```python
from build123d import *

# Parameters (mm, degrees)
F1_DEPTH    = 30
F2_W        = 1278
F2_H        = 510
F3_DEPTH    = 28
F4_W        = 500
F4_H        = 400
F5_DEPTH    = 300
F6_T        = 2
F6_T3_DEPTH = 34
F6_T5_DEPTH = 404
F6_T7_DEPTH = 504
F6_T9_DEPTH = 32
F7_R        = 50
F8_R        = 25
F9_DEPTH    = 2
F10_R       = 15
F10_R_2     = 20
F11_DEPTH   = 30
F12_W       = 510
F12_H       = 2
F13_DEPTH   = 5
F14_W       = 510
F14_H       = 2
F15_ANGLE   = 90
F16_W       = 2
F16_H       = 510
F17_DEPTH   = 10
F19_DEPTH   = 400
F20_R       = 150
F21_W       = 30
F21_H       = 30
F22_DEPTH   = 850
F23_W       = 30
F23_H       = 30
F24_DEPTH   = 1080
F25_W       = 30
F25_H       = 30
F26_DEPTH   = 480
F28_DEPTH   = 2


# Not quite as in the source:
# - a shell that OpenCascade refuses in one call is made with other operations: the cavity is built on its own and cut out


with BuildPart() as f1:
    # F0 (on Top) → F1 (new body)
    with BuildSketch(Plane.XY):
        Polygon((0, 690), (0, 0), (1280, 0), (1280, 725), (100, 725), (100, 690), align=None)
    extrude(amount=F1_DEPTH)

    # F2 (on face) → F3 (cut)
    with BuildSketch(Plane.XY.offset(30)):
        with Locations((641, 285)):
            Rectangle(F2_W, F2_H)
    extrude(amount=-F3_DEPTH, mode=Mode.SUBTRACT)

    # F4 (on face) → F5 (join)
    with BuildSketch(Plane(origin=(0, 0, 0), x_dir=(1, 0, 0), z_dir=(0, 0, -1))):
        with Locations((370, -285)):
            Rectangle(F4_W, F4_H)
    extrude(amount=F5_DEPTH)

    # F6: shell of thickness 2, made by hand


with BuildPart() as f6_core1:
    # F6_t2: copy of F1
    add(f1.part)

    # the walls: a layer under each face that stays
    f6_faces = [f6_core1.faces().sort_by_distance(p)[0] for p in [
        (0, 345, 15),
        (50, 690, 15),
        (640, 0, 15),
        (640, 362.5, 0),
        (213.3333333333, 604.1666666667, 30),
        (100, 707.5, 15),
        (1280, 604.1666666667, 25),
        (690, 725, 15),
        (620, 285, -150),
        (370, 485, -150),
        (120, 285, -150),
        (370, 85, -150),
        (641, 540, 16),
        (2, 285, 16),
        (641, 30, 16),
        (370, 285, -300),
    ]]
    thicken(f6_faces, amount=-F6_T, mode=Mode.SUBTRACT)

    # F6_s4 → F6_t3 (cut)
    with BuildSketch(Plane.XY.offset(-2)):
        Polygon((99.98, 690.02), (100, 688), (102, 688), (102, 690), align=None)
    extrude(amount=F6_T3_DEPTH, mode=Mode.SUBTRACT)

    # F6_s6 → F6_t5 (cut)
    with BuildSketch(Plane.XZ.offset(-487)):
        Polygon((620.02, -0.02), (620, 2), (618, 2), (618, 0), align=None)
        Polygon((119.98, -0.02), (120, 2), (122, 2), (122, 0), align=None)
    extrude(amount=F6_T5_DEPTH, mode=Mode.SUBTRACT)

    # F6_s8 → F6_t7 (cut)
    with BuildSketch(Plane.YZ.offset(118)):
        Polygon((485.02, -0.02), (485, 2), (483, 2), (483, 0), align=None)
        Polygon((84.98, -0.02), (85, 2), (87, 2), (87, 0), align=None)
    extrude(amount=F6_T7_DEPTH, mode=Mode.SUBTRACT)

    # F6_s10 → F6_t9 (cut)
    with BuildSketch(Plane.XY):
        Polygon((2.02, 539.98), (2, 542), (0, 542), (0, 540), align=None)
        Polygon((2.02, 30.02), (0, 30), (0, 28), (2, 28), align=None)
    extrude(amount=F6_T9_DEPTH, mode=Mode.SUBTRACT)


with BuildPart() as f1_1:
    add(f1.part)

    # what is left inside the walls is the cavity
    f6_cavity = [f6_core1.part.solids().sort_by_distance(p)[0] for p in [
        (640, 10.666667, 2.02),
        (640, 602.333333, 27.98),
        (370, 351, -297.98),
    ]]
    add(f6_cavity, mode=Mode.SUBTRACT)

    # F7
    f7_edges = [f1_1.edges().sort_by_distance(p)[0] for p in [
        (122, 483, -148),
        (618, 483, -148),
        (122, 87, -148),
        (618, 87, -148),
        (618, 285, -298),
        (370, 483, -298),
        (122, 285, -298),
        (370, 87, -298),
        (120, 85, -150),
        (370, 85, -300),
        (620, 85, -150),
        (620, 285, -300),
        (620, 485, -150),
        (370, 485, -300),
        (120, 485, -150),
        (120, 285, -300),
    ]]
    fillet(f7_edges, radius=F7_R)

    # F8 (on face) → F9 (cut, through all)
    with BuildSketch(Plane.XY.offset(-298)):
        with Locations((488, 353)):
            Circle(F8_R)
    extrude(amount=-F9_DEPTH, mode=Mode.SUBTRACT)

    # F10 (on face) → F11 (cut, through all)
    with BuildSketch(Plane.XY.offset(30)):
        with Locations((550, 632.5)):
            Circle(F10_R)
        with Locations((370, 632.5)):
            Circle(F10_R)
        with Locations((190, 632.5)):
            Circle(F10_R_2)
    extrude(amount=-F11_DEPTH, mode=Mode.SUBTRACT)

    # F12 (on face) → F13 (join)
    with BuildSketch(Plane.YZ.offset(1280)):
        with Locations((285, 1)):
            Rectangle(F12_W, F12_H)
    extrude(amount=F13_DEPTH)

    # F14 (on face) → F15 (revolve)
    with BuildSketch(Plane.YZ.offset(1285)):
        with Locations((285, 1)):
            Rectangle(F14_W, F14_H)
    revolve(axis=Axis((1285, 285, 0), (0, 1, 0)), revolution_arc=F15_ANGLE)

    # F16 (on face) → F17 (join)
    with BuildSketch(Plane(origin=(0, 0, 0), x_dir=(1, 0, 0), z_dir=(0, 0, -1))):
        with Locations((1286, -285)):
            Rectangle(F16_W, F16_H)
    extrude(amount=F17_DEPTH)

    # F18 (on face) → F19 (join)
    with BuildSketch(Plane.XY.offset(30)):
        Polygon((1278, 540), (1280, 540), (1280, 725), (100, 725), (100, 690), (0, 690), (0, 0), (2, 0), (2, 688), (102, 688), (102, 723), (1278, 723), align=None)
    extrude(amount=F19_DEPTH)

    # F20
    f20_edges = [f1_1.edges().sort_by_distance(p)[0] for p in [
        (1279, 540, 430),
        (1, 0, 430),
    ]]
    fillet(f20_edges, radius=F20_R)

    # F21 (on face) → F22 (join)
    with BuildSketch(Plane(origin=(0, 0, 0), x_dir=(1, 0, 0), z_dir=(0, 0, -1))):
        with Locations((85, -45)):
            Rectangle(F21_W, F21_H)
        with Locations((1195, -45)):
            Rectangle(F21_W, F21_H)
        with Locations((1195, -555)):
            Rectangle(F21_W, F21_H)
        with Locations((85, -555)):
            Rectangle(F21_W, F21_H)
    extrude(amount=F22_DEPTH)

    # F23 (on face) → F24 (join, through all)
    with BuildSketch(Plane.YZ.offset(100)):
        with Locations((45, -715)):
            Rectangle(F23_W, F23_H)
        with Locations((555, -715)):
            Rectangle(F23_W, F23_H)
    extrude(amount=F24_DEPTH)

    # F25 (on face) → F26 (join, through all)
    with BuildSketch(Plane(origin=(0, 60, 0), x_dir=(-1, 0, 0), z_dir=(0, 1, 0))):
        with Locations((-1195, -715)):
            Rectangle(F25_W, F25_H)
        with Locations((-85, -715)):
            Rectangle(F25_W, F25_H)
    extrude(amount=F26_DEPTH)

    # F27 (on face) → F28 (join)
    with BuildSketch(Plane.XY.offset(-700)):
        Polygon((100, 60), (100, 30), (1180, 30), (1180, 60), (1210, 60), (1210, 540), (1180, 540), (1180, 570), (100, 570), (100, 540), (70, 540), (70, 60), align=None)
    extrude(amount=F28_DEPTH)


solid = f1_1.part
```
Design review of the part built by this model. Coordinates are the model's own, in mm. A direction names the side the tool comes from. Give positions to 0.01 mm unless a question says otherwise; leave off trailing zeros. Order: outer loops, then holes, each group sorted by start corner. A loop starts at its lowest first (then second) coordinate and runs counter-clockwise, first axis right, second up. Notation, with made-up numbers: (39, 88) - (44, 88) arc R15 ccw to (44, 94) - close; hole circle Ø5 at (-11.5, 34). An arc over 180 degrees is marked (long way). Use a Markdown table: item, result. Add a question column.
(1) Clearance check with flat-ended pins moving along their axes: P1, Ø4, axis at x = 150.5, y = 406.5, coming from the +Z side; P2, Ø15, axis at y = 49, z = -769.5, coming from the +X side; P3, Ø7.5, axis at x = 1284, z = -5.5, coming from the -Y side. State where each tip first meets the part, or that it passes through.
(2) Machinability: for faces 5 (the face through (70, 541, -486)), 6 (the face through (643, 570, -710)), 7 (the face through (134.258, 469.964, -126.75)), 8 (the face through (1180, 45, -789)), 9 (the face through (794, 357, 0)), which of the approach directions +Z, -Z, +X, -X, +Y, -Y give a long, thin tool a straight path to every point of the face, cutting with its end or side? Answer none if there is none.
(3) Add section A-A on z = -62. Give the number of separate pieces and of enclosed holes in the cut face, then the cut area to 3 significant figures.
(4) Wall thickness on probe 1 along Y at (x, z) = (550, 29); probe 2 along X at (y, z) = (632, 1); probe 3 along Y at (x, z) = (190, 1): over which ranges is each line inside the solid? List them lowest first. Write a range as [from, to].
(5) Add section B-B on x = 1107. Give the boundary of the cut face in (y, z), then the cut area to 3 significant figures.
(6) Mouldability with a two-part tool opening along Z and no side actions: class faces 1 (the face through (372.772, 101.258, -282.964)), 2 (the face through (1195, 45, -850)), 3 (the face through (134.258, 282.9, -284.964)), 4 (the face through (51, 688, 227)) as +Z half, -Z half, draft (parallel to the pull), parting line (faces both ways), or undercut.
Report:
| question | item | result |
|---|---|---|
| 1 | P1 | stops at z = -292.13 |
| 1 | P2 | stops at x = 1210 |
| 1 | P3 | stops at y = 30 |
| 2 | face 5 | -Z, -X, +Y, -Y |
| 2 | face 6 | -Z, +X, -X, +Y |
| 2 | face 7 | -X, +Y |
| 2 | face 8 | -Z, +Y, -Y |
| 2 | face 9 | none |
| 3 | separate pieces | 5 |
| 3 | enclosed holes | 1 |
| 3 | area | 7,180 mm² |
| 4 | probe 1 | y = [0, 30], [540, 617.5], [647.5, 725] |
| 4 | probe 2 | x = [0, 170.01], [209.99, 355.01], [384.99, 535.01], [564.99, 1280] |
| 4 | probe 3 | y = [0, 87], [483, 612.5], [652.5, 725] |
| 5 | outline | (0, 0) - (725, 0) - (725, 430) - (723, 430) - (723, 30) - (540, 30) - (540, 2) - (30, 2) - (30, 30) - (0, 30) - close; (30, -730) - (60, -730) - (60, -700) - (540, -700) - (540, -730) - (570, -730) - (570, -698) - (30, -698) - close; hole (2, 2) - (28, 2) - (28, 28) - (2, 28) - close; hole (542, 2) - (723, 2) - (723, 28) - (542, 28) - close |
| 5 | area | 5,770 mm² |
| 6 | face 1 | +Z half |
| 6 | face 2 | -Z half |
| 6 | face 3 | undercut |
| 6 | face 4 | draft |
